Read the model definition and answer for the solid it produces. Units are mm, in the model's axes. Coordinates: 2 decimals unless noted, no trailing zeros. Write each loop counter-clockwise with the first axis right and the second up, starting at its lowest first coordinate (ties: lowest second). Pieces come first, ordered by that corner, then holes. Notation, with made-up numbers: (69.5, 10) - (104.5, 10) arc R26 cw to (104.5, 24) - close; hole circle Ø7 at (39, 69.5). An arc over 180 degrees is marked (long way). Use a Markdown table: item, result.
from build123d import *

# Parameters (mm, degrees)
SKETCH1_W                       = 152.4
SKETCH1_H                       = 76.2
BOSS_EXTRUDE1_DEPTH             = 6.35
TAP_DRILL_FOR_1_4_20_TAP1_D     = 5.1054
TAP_DRILL_FOR_1_4_20_TAP2_D     = 5.1054
TAP_DRILL_FOR_1_4_20_TAP2_DEPTH = 12.7
TAP_DRILL_FOR_1_4_20_TAP2_TIP   = 1.533816902
TAP_DRILL_FOR_1_4_20_TAP3_D     = 5.1054
TAP_DRILL_FOR_1_4_20_TAP3_DEPTH = 12.7
TAP_DRILL_FOR_1_4_20_TAP3_TIP   = 1.533816902


with BuildPart() as part:
    # Sketch1 → Boss-Extrude1 (new, symmetric)
    with BuildSketch(Plane(origin=(0, 0, 0), x_dir=(1, 0, 0), z_dir=(0, 1, 0))):
        Rectangle(SKETCH1_W, SKETCH1_H)
    extrude(amount=BOSS_EXTRUDE1_DEPTH, both=True)

    # Tap Drill for 1/4-20 Tap1 (through all)
    with Locations(Plane(origin=(0, 6.35, 0), x_dir=(1, 0, 0), z_dir=(0, 1, 0))):
        with Locations((63.5, 25.4), (38.1, 25.4), (12.7, 25.4), (38.1, 0), (12.7, 0), (38.1, -25.4), (12.7, -25.4), (63.5, 0), (63.5, -25.4), (-12.7, 25.4), (-38.1, 25.4), (-12.7, 0), (-38.1, 0), (-12.7, -25.4), (-38.1, -25.4)):
            Hole(TAP_DRILL_FOR_1_4_20_TAP1_D / 2)

    # Tap Drill for 1/4-20 Tap2
    with Locations(Plane.ZY.offset(76.2)):
        with Locations((-25.4, 0), (0, 0), (25.4, 0)):
            Hole(TAP_DRILL_FOR_1_4_20_TAP2_D / 2, depth=TAP_DRILL_FOR_1_4_20_TAP2_DEPTH)
            with Locations((0, 0, -(TAP_DRILL_FOR_1_4_20_TAP2_DEPTH + TAP_DRILL_FOR_1_4_20_TAP2_TIP / 2))):  # 118° drill point
                Cone(0, TAP_DRILL_FOR_1_4_20_TAP2_D / 2, TAP_DRILL_FOR_1_4_20_TAP2_TIP, mode=Mode.SUBTRACT)

    # Tap Drill for 1/4-20 Tap3
    with Locations(Plane(origin=(76.2, 0, 0), x_dir=(0, 0, -1), z_dir=(1, 0, 0))):
        with Locations((12.7, 0), (-12.7, 0)):
            Hole(TAP_DRILL_FOR_1_4_20_TAP3_D / 2, depth=TAP_DRILL_FOR_1_4_20_TAP3_DEPTH)
            with Locations((0, 0, -(TAP_DRILL_FOR_1_4_20_TAP3_DEPTH + TAP_DRILL_FOR_1_4_20_TAP3_TIP / 2))):  # 118° drill point
                Cone(0, TAP_DRILL_FOR_1_4_20_TAP3_D / 2, TAP_DRILL_FOR_1_4_20_TAP3_TIP, mode=Mode.SUBTRACT)


solid = part.part
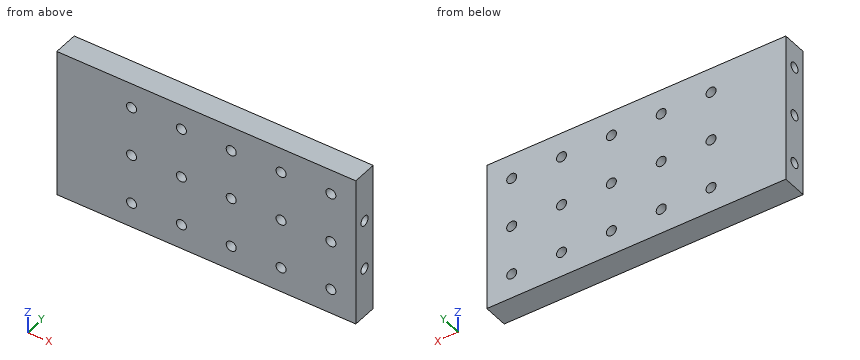
(1) Each of these flat-tipped pins is pushed along its axis until it touches: P1, Ø3, axis at y = 0, z = 12.7, coming from the +X side; P2, Ø6, axis at x = -12.7, z = -25.4, coming from the +Y side; P3, Ø4, axis at y = 0, z = -12.7, coming from the +X side. Where does it stop, or does it pass through?
Report:
| item | result |
|---|---|
| P1 | stops at x = 62.87 |
| P2 | stops at y = 6.35 |
| P3 | stops at x = 63.17 |
(2) A cutting plane is placed at B-B, the plane y = -4. Count the separate pieces of the cut face and the enclosed holes in it, and give its area (3 significant figures).
Report:
| item | result |
|---|---|
| separate pieces | 1 |
| enclosed holes | 15 |
| area | 11,300 mm² |
(3) A cutting plane is placed at A-A, the plane x = -38.1. Write down the section's boundary in (y, z).
Report:
| item | result |
|---|---|
| outline | (-6.35, -38.1) - (6.35, -38.1) - (6.35, -27.95) - (-6.35, -27.95) - close; (-6.35, -22.85) - (6.35, -22.85) - (6.35, -2.55) - (-6.35, -2.55) - close; (-6.35, 2.55) - (6.35, 2.55) - (6.35, 22.85) - (-6.35, 22.85) - close; (-6.35, 27.95) - (6.35, 27.95) - (6.35, 38.1) - (-6.35, 38.1) - close |
(4) Straight lines are drawn through the part: L1, parallel to Z at x = 12.7, y = -2.25; L2, parallel to X at y = -3, z = -25.4; L3, parallel to Z at x = 68.75, y = 0. For each, find the intervals that lie inside material, in ascending order.
Report:
| item | result |
|---|---|
| L1 | z = -38.1 to -27.95, -22.85 to -2.55, 2.55 to 22.85, 27.95 to 38.1 |
| L2 | x = -76.2 to -40.65, -35.55 to -15.25, -10.15 to 10.15, 15.25 to 35.55, 40.65 to 60.95, 66.05 to 76.2 |
| L3 | z = -38.1 to -15.25, -10.15 to 10.15, 15.25 to 38.1 |
